Print and shaded views of the part. All mm, measured from the part's lowest x, y and z. Coordinates: 2 decimals unless noted, no trailing zeros. Loops run counter-clockwise (first coordinate to the right, second up) from the corner with the lowest first, then second, coordinate; pieces in that order, holes last. Notation, with made-up numbers: (-30, -3) -> (9, -3) arc R17 cw to (9, 30) -> close; hole circle Ø1 at (61.25, -35). An arc over 180 degrees is marked (long way). One line per item, written item: value. Start each with the question number.
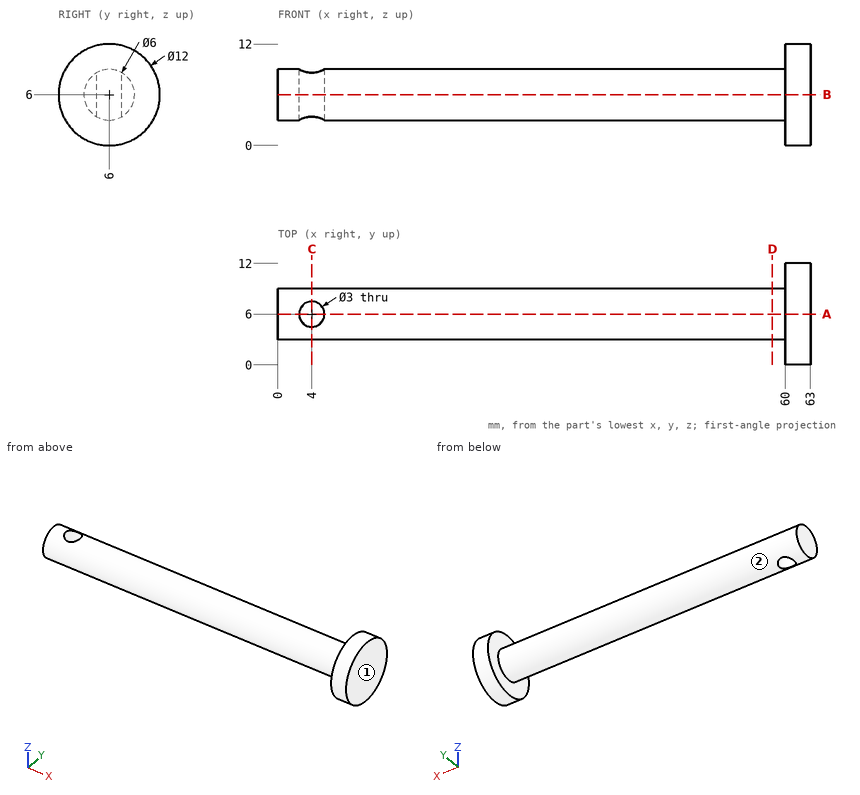
1) Slice it at D-D (x = 58.5). Give the cut face in (y, z), then the cut area to 3 significant figures.
2) Slice it at A-A (y = 6). Give the cut face in (x, z), then the cut area to 3 significant figures.
3) Pin check, flat tips, straight feed: pin 1 Ø4 at (x, y) = (22, 5) entering from -Z; pin 2 Ø1 at (x, y) = (15.5, 9) entering from +Z; pin 3 Ø3 at (x, y) = (34, 4) entering from +Z. Stop position of each tip, or through.
4) Probe line 1 (X direction, y = 6, z = 4.75); line 2 (Y direction, x = 4, z = 6.25); line 3 (X direction, y = 1, z = 7.75). List the from-to ranges inside material, lowest first. Write a range as from..to.
5) Pull direction Y, two halves, no side cores. Call the marked faces 1 and 2: +Y half, -Y half, draft (parallel to the pull), parting line (faces both ways), or undercut.
6) Slice it at B-B (z = 6). Give the cut face in (x, y).
7) Slice it at C-C (x = 4). Give the cut face in (y, z).
Check sheet entries:
1. outline: circle Ø6 at (6, 6)
1. area: 28.3 mm^2
2. outline: (0, 3) -> (2.5, 3) -> (2.5, 9) -> (0, 9) -> close; (5.5, 3) -> (60, 3) -> (60, 0) -> (63, 0) -> (63, 12) -> (60, 12) -> (60, 9) -> (5.5, 9) -> close
2. area: 378 mm^2
3. pin 1: stops at z = 3
3. pin 2: stops at z = 7.66
3. pin 3: stops at z = 8.96
4. line 1: x = 0..2.5, 5.5..63
4. line 2: y = 3.01..4.5, 7.5..8.99
4. line 3: x = 60..63
5. face 1: draft
5. face 2: parting line
6. outline: (0, 3) -> (60, 3) -> (60, 0) -> (63, 0) -> (63, 12) -> (60, 12) -> (60, 9) -> (0, 9) -> close; hole circle Ø3 at (4, 6)
7. outline: (4.5, 3.4) -> (4.5, 8.6) arc R3 ccw to start; (7.5, 3.4) arc R3 ccw to (7.5, 8.6) -> close
